from build123d import *

# Parameters (mm, degrees)
SK_SHROUD_W             = 48.72
SK_SHROUD_H             = 8.3
SHROUD_DEPTH            = 9.9
SK_FLANGE_EARS_W        = 3.4
SK_FLANGE_EARS_H        = 5.6
FLANGE_EARS_DEPTH       = 6
SK_CAVITY_W             = 46.72
SK_CAVITY_H             = 7.2
CAVITY_DEPTH            = 7.6
SK_TERMINAL_BLOCK_W     = 46.51
SK_TERMINAL_BLOCK_H     = 11.75
TERMINAL_BLOCK_DEPTH    = 10.1
INSERT_HOLES_DEPTH      = 34.295909659
INSERT_HOLES_DEPTH_BACK = 34.295909659
SK_INSERT_HOLES_R       = 1.25
SK_CONTACT_PINS_W       = 1
SK_CONTACT_PINS_H       = 1
CONTACT_PINS_DEPTH      = 6
SK_WIRE_ENTRIES_W       = 2.6
SK_WIRE_ENTRIES_H       = 2.8
WIRE_ENTRIES_DEPTH      = 6
SK_CLAMP_SCREW_HOLES_R  = 1.3
CLAMP_SCREW_HOLES_DEPTH = 3


with BuildPart() as part:
    # SK Shroud → Shroud (new body)
    with BuildSketch(Plane.XY.offset(3)):
        with Locations((0, -0.6)):
            Rectangle(SK_SHROUD_W, SK_SHROUD_H)
    extrude(amount=-SHROUD_DEPTH)

    # SK Flange ears → Flange ears (add)
    with BuildSketch(Plane.XY.offset(3)):
        with Locations((26.06, 0)):
            Rectangle(SK_FLANGE_EARS_W, SK_FLANGE_EARS_H)
        with Locations((-26.06, 0)):
            Rectangle(SK_FLANGE_EARS_W, SK_FLANGE_EARS_H)
    extrude(amount=-FLANGE_EARS_DEPTH)

    # SK Cavity → Cavity (cut)
    with BuildSketch(Plane.XY.offset(3)):
        with Locations((0, -0.6)):
            Rectangle(SK_CAVITY_W, SK_CAVITY_H)
    extrude(amount=-CAVITY_DEPTH, mode=Mode.SUBTRACT)

    # SK Terminal block → Terminal block (add)
    with BuildSketch(Plane.XY.offset(-6.9)):
        with Locations((0, 1.125)):
            Rectangle(SK_TERMINAL_BLOCK_W, SK_TERMINAL_BLOCK_H)
    extrude(amount=-TERMINAL_BLOCK_DEPTH)

    # SK Insert holes → Insert holes (cut, two sides: drawn at the far end of the back side and taken through both)
    with BuildSketch(Plane.XY.offset(-INSERT_HOLES_DEPTH_BACK)):
        with Locations((-25.375, 0)):
            Circle(SK_INSERT_HOLES_R)
        with Locations((25.375, 0)):
            Circle(SK_INSERT_HOLES_R)
    extrude(amount=INSERT_HOLES_DEPTH + INSERT_HOLES_DEPTH_BACK, mode=Mode.SUBTRACT)

    # SK Contact pins → Contact pins (add)
    with BuildSketch(Plane.XY.offset(-4.6)):
        with Locations((-20.955, -0.6)):
            Rectangle(SK_CONTACT_PINS_W, SK_CONTACT_PINS_H)
        with Locations((-17.145, -0.6)):
            Rectangle(SK_CONTACT_PINS_W, SK_CONTACT_PINS_H)
        with Locations((-13.335, -0.6)):
            Rectangle(SK_CONTACT_PINS_W, SK_CONTACT_PINS_H)
        with Locations((-9.525, -0.6)):
            Rectangle(SK_CONTACT_PINS_W, SK_CONTACT_PINS_H)
        with Locations((-5.715, -0.6)):
            Rectangle(SK_CONTACT_PINS_W, SK_CONTACT_PINS_H)
        with Locations((-1.905, -0.6)):
            Rectangle(SK_CONTACT_PINS_W, SK_CONTACT_PINS_H)
        with Locations((1.905, -0.6)):
            Rectangle(SK_CONTACT_PINS_W, SK_CONTACT_PINS_H)
        with Locations((5.715, -0.6)):
            Rectangle(SK_CONTACT_PINS_W, SK_CONTACT_PINS_H)
        with Locations((9.525, -0.6)):
            Rectangle(SK_CONTACT_PINS_W, SK_CONTACT_PINS_H)
        with Locations((13.335, -0.6)):
            Rectangle(SK_CONTACT_PINS_W, SK_CONTACT_PINS_H)
        with Locations((17.145, -0.6)):
            Rectangle(SK_CONTACT_PINS_W, SK_CONTACT_PINS_H)
        with Locations((20.955, -0.6)):
            Rectangle(SK_CONTACT_PINS_W, SK_CONTACT_PINS_H)
    extrude(amount=CONTACT_PINS_DEPTH)

    # SK Wire entries → Wire entries (cut)
    with BuildSketch(Plane.XY.offset(-17)):
        with Locations((-20.955, -2)):
            Rectangle(SK_WIRE_ENTRIES_W, SK_WIRE_ENTRIES_H)
        with Locations((-17.145, -2)):
            Rectangle(SK_WIRE_ENTRIES_W, SK_WIRE_ENTRIES_H)
        with Locations((-13.335, -2)):
            Rectangle(SK_WIRE_ENTRIES_W, SK_WIRE_ENTRIES_H)
        with Locations((-9.525, -2)):
            Rectangle(SK_WIRE_ENTRIES_W, SK_WIRE_ENTRIES_H)
        with Locations((-5.715, -2)):
            Rectangle(SK_WIRE_ENTRIES_W, SK_WIRE_ENTRIES_H)
        with Locations((-1.905, -2)):
            Rectangle(SK_WIRE_ENTRIES_W, SK_WIRE_ENTRIES_H)
        with Locations((1.905, -2)):
            Rectangle(SK_WIRE_ENTRIES_W, SK_WIRE_ENTRIES_H)
        with Locations((5.715, -2)):
            Rectangle(SK_WIRE_ENTRIES_W, SK_WIRE_ENTRIES_H)
        with Locations((9.525, -2)):
            Rectangle(SK_WIRE_ENTRIES_W, SK_WIRE_ENTRIES_H)
        with Locations((13.335, -2)):
            Rectangle(SK_WIRE_ENTRIES_W, SK_WIRE_ENTRIES_H)
        with Locations((17.145, -2)):
            Rectangle(SK_WIRE_ENTRIES_W, SK_WIRE_ENTRIES_H)
        with Locations((20.955, -2)):
            Rectangle(SK_WIRE_ENTRIES_W, SK_WIRE_ENTRIES_H)
    extrude(amount=WIRE_ENTRIES_DEPTH, mode=Mode.SUBTRACT)

    # SK Clamp screw holes → Clamp screw holes (cut)
    with BuildSketch(Plane(origin=(0, 7, 0), x_dir=(1, 0, 0), z_dir=(0, 1, 0))):
        with Locations(Location((-20.955, 12, 0), (0, 0, 270))):
            Circle(SK_CLAMP_SCREW_HOLES_R)
        with Locations(Location((-17.145, 12, 0), (0, 0, 270))):
            Circle(SK_CLAMP_SCREW_HOLES_R)
        with Locations(Location((-13.335, 12, 0), (0, 0, 270))):
            Circle(SK_CLAMP_SCREW_HOLES_R)
        with Locations(Location((-9.525, 12, 0), (0, 0, 270))):
            Circle(SK_CLAMP_SCREW_HOLES_R)
        with Locations(Location((-5.715, 12, 0), (0, 0, 270))):
            Circle(SK_CLAMP_SCREW_HOLES_R)
        with Locations(Location((-1.905, 12, 0), (0, 0, 270))):
            Circle(SK_CLAMP_SCREW_HOLES_R)
        with Locations(Location((1.905, 12, 0), (0, 0, 270))):
            Circle(SK_CLAMP_SCREW_HOLES_R)
        with Locations(Location((5.715, 12, 0), (0, 0, 270))):
            Circle(SK_CLAMP_SCREW_HOLES_R)
        with Locations(Location((9.525, 12, 0), (0, 0, 270))):
            Circle(SK_CLAMP_SCREW_HOLES_R)
        with Locations(Location((13.335, 12, 0), (0, 0, 270))):
            Circle(SK_CLAMP_SCREW_HOLES_R)
        with Locations(Location((17.145, 12, 0), (0, 0, 270))):
            Circle(SK_CLAMP_SCREW_HOLES_R)
        with Locations(Location((20.955, 12, 0), (0, 0, 270))):
            Circle(SK_CLAMP_SCREW_HOLES_R)
    extrude(amount=-CLAMP_SCREW_HOLES_DEPTH, mode=Mode.SUBTRACT)


solid = part.part
The model under review builds one solid part; all positions refer to its coordinate system, in mm. A direction names the side the tool comes from. Round coordinates to 2 decimals unless told otherwise and drop trailing zeros. Loops run counter-clockwise (first coordinate to the right, second up) from the corner with the lowest first, then second, coordinate; pieces in that order, holes last. Notation, with made-up numbers: (-37, -12.5) -> (-6, -12.5) arc R13 cw to (-6, 8.5) -> close; hole circle Ø8 at (-5, -14.5). An arc over 180 degrees is marked (long way). Return JSON: item names as keys, results as strings.
(1) For pin 1 (3 mm diameter, centred on x = 20.5, y = -2, fed in from +Z); pin 2 (0.8 mm diameter, centred on x = 16.5, z = -12, fed in from +Y); pin 3 (2 mm diameter, centred on x = -1, z = -4, fed in from +Y), all flat-tipped, find the tip position at first contact; note any pin that passes through.
Solved:
{"pin 1": "z = 1.4", "pin 2": "y = 4", "pin 3": "y = 3.55"}
(2) Add section A-A on y = 2.25. Write out the cut boundary in (x, z) (3 decimals), plus the area to 3 significant figures.
Solved:
{"outline": "(-27.76, -3) -> (-24.36, -3) -> (-24.36, -6.9) -> (-23.255, -6.9) -> (-23.255, -17) -> (23.255, -17) -> (23.255, -6.9) -> (24.36, -6.9) -> (24.36, -3) -> (27.76, -3) -> (27.76, 3) -> (23.36, 3) -> (23.36, -4.6) -> (-23.36, -4.6) -> (-23.36, 3) -> (-27.76, 3) -> close", "area": "638 mm2"}
(3) The part is to be moulded in two halves that separate along Z. For faces 3 (the flat face through (-10, 4, -12)), 4 (the flat face through (-9.5, -0.1, -1.6)), 5 (the flat face through (-0.1, -4.6, 3)), say which applies: released by +Z, released by -Z, zero draft, split by the parting line, or undercut.
Solved:
{"face 3": "undercut", "face 4": "zero draft", "face 5": "released by +Z"}
(4) For line 1 (Y direction, x = 2.5, z = -0.5); line 2 (Y direction, x = 6, z = 0); line 3 (Y direction, x = 1, z = -15.25), list the stretches that pass through material, from the lowest coordinate up.
Solved:
{"line 1": "-4.75 to -4.2, 3 to 3.55", "line 2": "-4.75 to -4.2, -1.1 to -0.1, 3 to 3.55", "line 3": "-4.75 to -3.4, -0.6 to 7"}
(5) Add section C-C on z = -0.5. State how many separate pieces and enclosed holes the cut face has, plus the area to 3 significant figures.
Solved:
{"separate pieces": "13", "enclosed holes": "3", "area": "108 mm2"}
(6) For faces 1 (the flat face through (-6.215, -0.6, -1.6)), 2 (the flat face through (0.605, -2, -14)), list the 3-axis set-ups (+Z, -Z, +X, -X, +Y, -Y) from which the entire face can be reached by the end or side of a thin tool; tool diameter is ignored.
Solved:
{"face 1": "+Z", "face 2": "-Z"}
(7) Add section B-B on z = -5.75. Write out the cut boundary in (x, y) (3 decimals), plus the area to 3 significant figures.
Solved:
{"outline": "(-24.36, -4.75) -> (24.36, -4.75) -> (24.36, -0.73) arc R1.25 cw to (24.36, 0.73) -> (24.36, 3.55) -> (-24.36, 3.55) -> (-24.36, 0.73) arc R1.25 cw to (-24.36, -0.73) -> close", "area": "404 mm2"}
